For this review, take the finished solid that the model builds, in its own axes (mm). A direction names the side the tool comes from. Give positions to 0.01 mm unless a question says otherwise; leave off trailing zeros. Order: outer loops, then holes, each group sorted by start corner. A loop starts at its lowest first (then second) coordinate and runs counter-clockwise, first axis right, second up. Notation, with made-up numbers: M 21.5,24.5 L 56.5,24.5 A27 cw 56.5,63.5 Z; hole C 17.25,-27.75 d3. An arc over 180 degrees is marked long. Use CSV: the item, a comma, the result in double quotes. Start each with the question number.
(1) Wall thickness on L1, parallel to X at y = -4.75, z = 0; L2, parallel to X at y = -2.7, z = 0; L3, parallel to X at y = -4.3, z = 2.75: over which ranges is each line inside the solid? List them lowest first. Write a range as from..to.
(2) Consider section B-B (z = 0). Write out the cut boundary in (x, y).
(3) Draft analysis for pull direction Z (two halves, no side actions). For faces 1 (the face through (-3, 0, 3)), 2 (the face through (-7.81, -2.54, 1.73)), 3 (the face through (4.3, -4.85, -2.74)), state which applies: pulls with the +Z half, pulls with the -Z half, needs draft (parallel to the pull), parting line crosses it, or undercut.
(4) Consider section A-A (x = 0). Write out the cut boundary in (y, z).
(5) Tool access review of faces 4 (the face through (5, -0.3, 2)), 5 (the face through (-3, -5, 3)), 6 (the face through (-2.16, -4.85, -6.87)): name each direction out of +Z, -Z, +X, -X, +Y, -Y from which nothing blocks a thin tool from reaching the whole face with its end or side.
(6) Consider section C-C (y = -1.45). Write out the cut boundary in (x, z).
(7) Consider section D-D (z = -6.25). Write out the cut boundary in (x, y).
(8) Clearance check with flat-ended pins moving along their axes: P1, Ø1, axis at y = -2.5, z = -5, coming from the -X side; P2, Ø1, axis at y = -2.5, z = 5.5, coming from the +X side (3 decimals); P3, Ø1, axis at y = -1.5, z = 1.5, coming from the +X side. State where each tip first meets the part, or that it passes through.
Autodesk Inventor part; units mm, degrees
ref_plane "YZ Plane" through (0, 0, 0) normal (1, 0, 0) x (0, 1, 0)
ref_plane "XZ Plane" through (0, 0, 0) normal (0, 1, 0) x (-1, 0, 0)
ref_plane "XY Plane" through (0, 0, 0) normal (0, 0, 1) x (1, 0, 0)
sketch "Sketch1" plane through (0, 0, 0) normal (1, 0, 0) x (0, 1, 0)
  line L0 (-5, -4.25) -> (-5, -5.9)
  line L1 (0, -4) -> (0, -5.1)
  line L2 (0, -5.1) -> (-0.3, -5.1)
  line L3 (-0.3, -5.1) -> (-0.3, -7.2)
  line L4 (-0.3, -7.2) -> (0, -7.2)
  line L5 (0, -7.2) -> (0, -8)
  line L6 (0, -8) -> (-5, -8)
  line L7 (-5, -8) -> (-5, -7.2)
  line L8 (-5, -7.2) -> (-4.7, -7.2)
  line L9 (-4.7, -7.2) -> (-4.7, -5.1)
  line L10 (-4.7, -5.1) -> (-5, -5.1)
  line L11 (-5, -5.1) -> (-5, -4)
  line L12 (-5, -4) -> (0, -4)
  line L13 (0, 0) -> (-5.2831, 0)
revolve "Revolution1" add sketch "Sketch1" angle 360 about axis through (0, 0, 0) along (0, -1, 0)
properties part number "Ball Bearing 8 x 16 x 5" material "Stainless Steel"
Check result:
1,L1,"x = -8..-7.2, -5.1..-4, 4..5.1, 7.2..8"
1,L2,"x = -8..-4, 4..8"
1,L3,"x = -7.51..-2.9, 2.9..7.51"
2,outline,"M -8,-5 L -7.2,-5 L -7.2,-4.7 L -5.1,-4.7 L -5.1,-5 L -4,-5 L -4,0 L -5.1,0 L -5.1,-0.3 L -7.2,-0.3 L -7.2,0 L -8,0 Z; M 4,-5 L 5.1,-5 L 5.1,-4.7 L 7.2,-4.7 L 7.2,-5 L 8,-5 L 8,0 L 7.2,0 L 7.2,-0.3 L 5.1,-0.3 L 5.1,0 L 4,0 Z"
3,face 1,"needs draft"
3,face 2,"parting line crosses it"
3,face 3,"undercut"
4,outline,"M -5,-8 L 0,-8 L 0,-7.2 L -0.3,-7.2 L -0.3,-5.1 L 0,-5.1 L 0,-4 L -5,-4 L -5,-5.1 L -4.7,-5.1 L -4.7,-7.2 L -5,-7.2 Z; M -5,4 L 0,4 L 0,5.1 L -0.3,5.1 L -0.3,7.2 L 0,7.2 L 0,8 L -5,8 L -5,7.2 L -4.7,7.2 L -4.7,5.1 L -5,5.1 Z"
5,face 4,"+Y"
5,face 5,"+Z, -Z, +X, -X, -Y"
5,face 6,"-Y"
6,outline,"C 0,0 d16; hole C 0,0 d8"
7,outline,"M -4.99,-5 L -3.57,-5 L -3.57,-4.7 L 3.57,-4.7 L 3.57,-5 L 4.99,-5 L 4.99,0 L 3.57,0 L 3.57,-0.3 L -3.57,-0.3 L -3.57,0 L -4.99,0 Z"
8,P1,"stops at x = -6.61"
8,P2,"stops at x = 6.245"
8,P3,"stops at x = 7.94"
